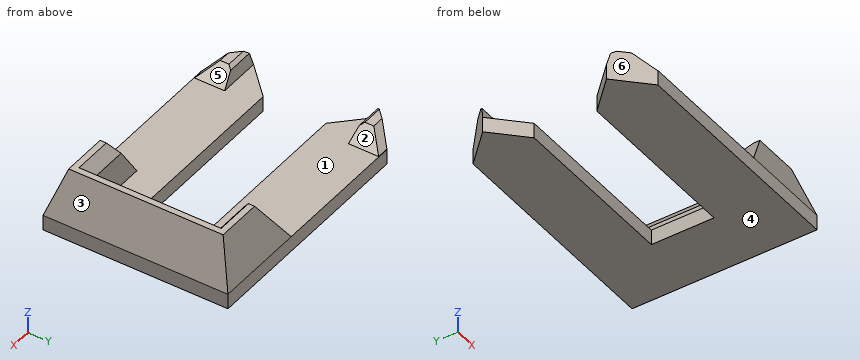
```python
from build123d import *

# Parameters (mm, degrees)
F0_W           = 172
F0_H           = 60.5
F4_DEPTH       = 5
F6_SIZE2       = 4
F6_SIZE        = 3
F9_DEPTH       = 5
F10_SIZE       = 4.99999
F11_SIZE2      = 0.99999
F11_SIZE       = 4.99999
F12_SIZE       = 1
F14_W          = 132
F14_H          = 20.5
F15_DEPTH      = 12.5
F17_DEPTH      = 25
F17_DEPTH_BACK = 25


# Not quite as in the source:
# - a fillet or chamfer is up to 0.001 mm smaller than in the source, because OpenCascade refuses the exact size


with BuildPart() as f4:
    # F0 (on Top) → F4 (new body)
    with BuildSketch(Plane.XY):
        Rectangle(F0_W, F0_H)
    extrude(amount=-F4_DEPTH)

    # F3 (on Top) → F5 section 0
    with BuildSketch(Plane.XY):
        Polygon((-86, 0), (-86, -30.25), (-55.75, -30.25), (-55.75, -20.25), (-76, -20.25), (-76, 0), align=None)
    # F2 (on offset) → F5 section 1
    with BuildSketch(Plane.XY.offset(15)):
        Polygon((-76, -20.25), (-76, 0), (-81, 0), (-81, -25.25), (-66, -25.25), (-66, -20.25), align=None)
    loft()

    # F6
    f6_edges = [f4.edges().sort_by_distance(p)[0] for p in [
        (-76, -10.125, 15),
        (-71, -20.25, 15),
    ]]
    chamfer(f6_edges, length=F6_SIZE, length2=F6_SIZE2)

    # F7: F4 across plane


with BuildPart() as f4_1:
    add(f4.part)
    add(f4.part.mirror(Plane.YZ))

    # F8 (on face) → F9 (join)
    with BuildSketch(Plane.XY):
        Polygon((13.8189587742, -20.25), (0, -20.25), (-13.8189587742, -20.25), (-13.8189587742, -30.1344580948), (0, -30.1344580948), (13.8189587742, -30.1344580948), align=None)
    extrude(amount=F9_DEPTH)

    # F10 (size 5 in the source; OpenCascade refuses exactly that, so slightly less here)
    f10_edges = [f4_1.edges().sort_by_distance(p)[0] for p in [
        (13.818959, -25.192229, 5),
        (0, -30.134458, 5),
        (-13.818959, -25.192229, 5),
    ]]
    chamfer(f10_edges, length=F10_SIZE)

    # F11 (size 5 and 1 in the source; OpenCascade refuses exactly that, so slightly less here)
    f11_edges = [f4_1.edges().sort_by_distance(p)[0] for p in [
        (0, -20.25, 5),
    ]]
    f11_side = f4_1.faces().sort_by_distance((0, -20.25, 2.315943))[0]
    chamfer(f11_edges, length=F11_SIZE, length2=F11_SIZE2, reference=f11_side)

    # F12
    f12_edges = [f4_1.edges().sort_by_distance(p)[0] for p in [
        (0, -21.24999, 5),
    ]]
    chamfer(f12_edges, length=F12_SIZE)

    # F13: F4 across plane


with BuildPart() as f4_2:
    add(f4_1.part)
    add(f4_1.part.mirror(Plane.XZ))

    # F14 (on Top) → F15 (cut, symmetric)
    with BuildSketch(Plane.XY):
        Rectangle(F14_W, F14_H)
    extrude(amount=F15_DEPTH, both=True, mode=Mode.SUBTRACT)


with BuildPart() as f17:
    # F16 (on Top) → F17 (new body, two sides)
    with BuildSketch(Plane.XY) as f17_sk:
        Polygon((23.7979591321, 44.0479591321), (0, 20.25), (18.644013716, 1.605986284), (18.644013716, -1.605986284), (0, -20.25), (26.894013716, -47.144013716), (91.0670285058, -47.144013716), (91.0670285058, 44.0479591321), align=None)
    extrude(amount=F17_DEPTH)
    extrude(f17_sk.sketch, amount=-F17_DEPTH_BACK)

    # F18: intersect F4
    add(f4_2.part, mode=Mode.INTERSECT)


solid = f17.part
```
The model under review builds one solid part; all positions refer to its coordinate system, in mm. Face numbers are marked on the shaded views. A direction names the side the tool comes from. Round coordinates to 2 decimals unless told otherwise and drop trailing zeros. Loops run counter-clockwise (first coordinate to the right, second up) from the corner with the lowest first, then second, coordinate; pieces in that order, holes last.
Item 1: Take a section at C-C (y = -3). Write out the cut boundary in (x, z), then the cut area to 4 significant figures.
Determined:
outline: (66, -5) - (86, -5) - (86, 0) - (81, 15) - (79, 15) - (76, 11) - (76, 0) - (66, 0) - close
area: 206.5 mm2
Item 2: Clearance check with flat-ended pins moving along their axes: pin 1 Ø8 at (y, z) = (23.5, 12.5) entering from +X; pin 2 Ø0.9 at (x, y) = (4.5, 23.5) entering from +Z; pin 3 Ø5.5 at (y, z) = (7.5, 5) entering from -X. State where each tip first meets the part, or that it passes through.
Determined:
pin 1: stops at x = 83.17
pin 2: stops at z = 5
pin 3: stops at x = 76
Item 3: Mouldability with a two-part tool opening along X and no side actions: class the marked faces 4, 5 and 6 as released by +X, released by -X, zero draft, split by the parting line, or undercut.
Determined:
face 4: zero draft
face 5: undercut
face 6: released by -X
Item 4: Take a section at A-A (y = -12.5). Write out the cut boundary in (x, z), then the cut area to 3 significant figures.
Determined:
outline: (7.75, -5) - (86, -5) - (86, 0) - (81, 15) - (79, 15) - (76, 11) - (76, 0) - (7.75, 0) - close
area: 498 mm2
Item 5: For line 1 (Y direction, x = 39, z = -3.25); line 2 (X direction, y = 0, z = -0.5); line 3 (Z direction, x = 43.5, y = 12), list the stretches that pass through material, from the lowest coordinate up.
Determined:
line 1: y = -30.25 to -10.25, 10.25 to 30.25
line 2: x = 66 to 86
line 3: z = -5 to 0
Item 6: For the marked faces 1, 2 and 3, list the 3-axis set-ups (+Z, -Z, +X, -X, +Y, -Y) from which the entire face can be reached by the end or side of a thin tool; tool diameter is ignored.
Determined:
face 1: +Z
face 2: +Z, +Y, -Y
face 3: +Z, +X, +Y, -Y
Item 7: Take a section at B-B (x = 45). Write out the cut boundary in (y, z).
Determined:
outline: (-30.25, -5) - (-10.25, -5) - (-10.25, 0) - (-30.25, 0) - close; (10.25, -5) - (30.25, -5) - (30.25, 0) - (10.25, 0) - close
